from build123d import *

# Parameters (mm, degrees)
BOSS_EXTRUDE1_DEPTH     = 15
CUT_EXTRUDE1_DEPTH      = 3.9
SKETCH4_R               = 1.75
CUT_EXTRUDE2_DEPTH      = 108.462598145
CUT_EXTRUDE3_DEPTH      = 108.935165725
CUT_EXTRUDE3_DEPTH_BACK = 108.935165725
CUT_EXTRUDE5_DEPTH      = 108.935165725


with BuildPart() as part:
    # Sketch2 → Boss-Extrude1 (new body)
    with BuildSketch(Plane.YZ):
        with BuildLine():
            Line((54.106158457, 5), (100, 5))
            ThreePointArc((100, 5), (105, 0), (100, -5))
            Line((100, -5), (54.106158457, -5))
            ThreePointArc((54.106158457, -5), (40.214304243, -6.215379759), (26.744546991, -9.824590337))
            Line((26.744546991, -9.824590337), (23.135674536, -11.13811249))
            ThreePointArc((23.135674536, -11.13811249), (16.479451078, -13.906430601), (10.0994572, -17.262704431))
            ThreePointArc((10.0994572, -17.262704431), (-20, 0), (10.0994572, 17.262704431))
            ThreePointArc((10.0994572, 17.262704431), (16.479451078, 13.906430601), (23.135674536, 11.13811249))
            Line((23.135674536, 11.13811249), (26.744546991, 9.824590337))
            ThreePointArc((26.744546991, 9.824590337), (40.214304243, 6.215379759), (54.106158457, 5))
        make_face()
        with BuildLine():
            Line((45, 3), (100, 3))
            ThreePointArc((100, 3), (103, 0), (100, -3))
            Line((100, -3), (45, -3))
            ThreePointArc((45, -3), (42, 0), (45, 3))
        make_face(mode=Mode.SUBTRACT)
    extrude(amount=-BOSS_EXTRUDE1_DEPTH)

    # Sketch3 → Cut-Extrude1 (cut)
    with BuildSketch(Plane.YZ):
        with BuildLine():
            Line((24.33053856, 3.5), (12, 3.5))
            ThreePointArc((12, 3.5), (8.440790603, 3.996719292), (5.153570125, 5.448918697))
            ThreePointArc((5.153570125, 5.448918697), (-7.5, 0), (5.153570125, -5.448918697))
            ThreePointArc((5.153570125, -5.448918697), (8.440790603, -3.996719292), (12, -3.5))
            Line((12, -3.5), (24.33053856, -3.5))
            ThreePointArc((24.33053856, -3.5), (27.83053856, 0), (24.33053856, 3.5))
        make_face()
    extrude(amount=-CUT_EXTRUDE1_DEPTH, mode=Mode.SUBTRACT)

    # Sketch4 → Cut-Extrude2 (cut, through all)
    with BuildSketch(Plane.YZ.offset(-3.9)):
        with Locations(Location((20, 0, 0), (0, 0, 270))):
            Circle(SKETCH4_R)
        with Locations(Location((24, 0, 0), (0, 0, 270))):
            Circle(SKETCH4_R)
        with Locations(Location((0, 0, 0), (0, 0, 270))):
            Circle(SKETCH4_R)
    extrude(amount=-CUT_EXTRUDE2_DEPTH, mode=Mode.SUBTRACT)

    # Sketch5 → Cut-Extrude3 (cut, two sides: drawn at the far end of the back side and taken through both)
    with BuildSketch(Plane(origin=(0, 0, 0), x_dir=(0, 1, 0), z_dir=(0, 0, 1)).offset(-CUT_EXTRUDE3_DEPTH_BACK)):
        Polygon((30, 15), (105, 11.069416554), (105, 15), align=None)
        Polygon((105, 0), (105, 3.930583446), (30, 0), align=None)
    extrude(amount=CUT_EXTRUDE3_DEPTH + CUT_EXTRUDE3_DEPTH_BACK, mode=Mode.SUBTRACT)

    # Sketch8 → Cut-Extrude5 (cut, through all)
    with BuildSketch(Plane.YZ):
        with BuildLine():
            ThreePointArc((11.490666647, 9.641814145), (-15, 0), (11.490666647, -9.641814145))
            ThreePointArc((11.490666647, -9.641814145), (11.182524563, -6.119734013), (7.660444431, -6.427876097))
            ThreePointArc((7.660444431, -6.427876097), (-10, 0), (7.660444431, 6.427876097))
            ThreePointArc((7.660444431, 6.427876097), (11.182524563, 6.119734013), (11.490666647, 9.641814145))
        make_face()
    extrude(amount=-CUT_EXTRUDE5_DEPTH, mode=Mode.SUBTRACT)


solid = part.part
The model under review builds one solid part; all positions refer to its coordinate system, in mm. A direction names the side the tool comes from. Coordinates: 2 decimals unless noted, no trailing zeros. Write each loop counter-clockwise with the first axis right and the second up, starting at its lowest first coordinate (ties: lowest second). Pieces come first, ordered by that corner, then holes. Notation, with made-up numbers: (-34.5, -5.5) - (19.5, -5.5) arc R17 ccw to (19.5, 0.5) - close; hole circle Ø2 at (1, 34). An arc over 180 degrees is marked (long way). Answer as a JSON object with one key per item and string values. Group by question number.
1. Mouldability with a two-part tool opening along Z and no side actions: class faces 4 (the face through (-7.4, -19.99, -0.59)), 5 (the face through (-7, 42, 0)), 6 (the face through (-7.4, 40.41, -6.18)) as pulls with the +Z half, pulls with the -Z half, needs draft (parallel to the pull), parting line crosses it, or undercut.
2. Add section B-B (y = 47). Give the boundary of the cut face in (x, z), plus the area to 3 significant figures.
3. Add section C-C (z = -13). Give the boundary of the cut face in (x, y), plus the area to 3 significant figures.
4. Clearance check with flat-ended pins moving along their axes: pin 1 Ø3 at (x, y) = (-1.5, 19.5) entering from +Z; pin 2 Ø3 at (x, y) = (-8.5, 48) entering from +Z; pin 3 Ø8 at (x, y) = (-11.5, 26) entering from -Z; pin 4 Ø24 at (y, z) = (0, 0) entering from -X. State where each tip first meets the part, or that it passes through.
5. Machinability: for faces 1 (the face through (-7, 77, 5)), 2 (the face through (-7, 103, 0)), 3 (the face through (-1.92, 8.39, -4.01)), which of the approach directions +Z, -Z, +X, -X, +Y, -Y give a long, thin tool a straight path to every point of the face, cutting with its end or side? Answer none if there is none.
6. Add section A-A (y = 0). Give the boundary of the cut face in (x, z).
7. Add section D-D (z = 0). Give the number of separate pieces and of enclosed holes in the cut face, plus the area to 3 significant figures.
8. To check wall thickness, follow probe 1 along Y at (x, z) = (-8.25, 0); probe 2 along Z at (x, y) = (-11.5, 66); probe 3 along Z at (x, y) = (-1.6, 0). State the ranges of each line that lie inside material, in increasing order.
Findings:
{
 "1": {"face 4": "parting line crosses it", "face 5": "undercut", "face 6": "pulls with the -Z half"},
 "2": {"outline": "(-14.11, -5.32) - (-0.89, -5.32) - (-0.89, -3) - (-14.11, -3) - close; (-14.11, 3) - (-0.89, 3) - (-0.89, 5.32) - (-14.11, 5.32) - close", "area": "61.2 mm²"},
 "3": {"outline": "(-15, -15.2) - (0, -15.2) - (0, -7.48) - (-15, -7.48) - close; (-15, 7.48) - (0, 7.48) - (0, 18.48) - (-15, 18.48) - close", "area": "281 mm²"},
 "4": {"pin 1": "z = 13.21", "pin 2": "z = 5.36", "pin 3": "z = -11.56", "pin 4": "x = -15"},
 "5": {"face 1": "+Z, +X, -X, +Y", "face 2": "+X, -X", "face 3": "+X"},
 "6": {"outline": "(-15, -20) - (0, -20) - (0, -15) - (-15, -15) - close; (-15, -10) - (0, -10) - (0, -7.5) - (-3.9, -7.5) - (-3.9, -1.75) - (-15, -1.75) - close; (-15, 1.75) - (-3.9, 1.75) - (-3.9, 7.5) - (0, 7.5) - (0, 10) - (-15, 10) - close; (-15, 15) - (0, 15) - (0, 20) - (-15, 20) - close"},
 "7": {"separate pieces": "6", "enclosed holes": "0", "area": "608 mm²"},
 "8": {"probe 1": "-20 to -15, -10 to -1.75, 1.75 to 18.25, 21.75 to 22.25, 25.75 to 42, 103 to 105", "probe 2": "-5 to -3, 3 to 5", "probe 3": "-20 to -15, -10 to -7.5, 7.5 to 10, 15 to 20"}
}
